Could you check a few things on this model? Use its own coordinates, in mm. A direction names the side the tool comes from. Round coordinates to 2 decimals unless told otherwise and drop trailing zeros. Loops run counter-clockwise (first coordinate to the right, second up) from the corner with the lowest first, then second, coordinate; pieces in that order, holes last. Notation, with made-up numbers: (-19, -2.5) - (-3, -2.5) arc R18 ccw to (-3, 31.5) - close; hole circle Ø10 at (57.25, 86.5). An arc over 180 degrees is marked (long way). Use one line per item in the form item = value.
```python
from build123d import *

# Parameters (mm, degrees)
F0_W      = 30
F0_H      = 22
F1_DEPTH  = 5
F2_DEPTH  = 39.1
F3_W      = 30
F3_H      = 12.7
F4_DEPTH  = 50
F8_W      = 30
F8_H      = 5
F9_DEPTH  = 25
F10_W     = 30
F10_H     = 5
F11_DEPTH = 5
F12_W     = 30
F12_H     = 5
F13_DEPTH = 25
F15_DEPTH = 25
F16_DEPTH = 3
F18_DEPTH = 3
F19_DEPTH = 3
F21_DEPTH = 3
F23_DEPTH = 30
F24_R     = 2.75
F25_DEPTH = 500
F26_W     = 68.0921077728
F26_H     = 72.8289508261
F27_DEPTH = 25
F29_DEPTH = 36
F30_R     = 4.99999
F32_DEPTH = 1
F33_W     = 82.302633673
F33_H     = 75.4934260622
F34_DEPTH = 50


# Not quite as in the source:
# - a fillet or chamfer is up to 0.001 mm smaller than in the source, because OpenCascade refuses the exact size


with BuildPart() as f1:
    # F0 (on Front) → F1 (new body)
    with BuildSketch(Plane.XZ):
        with Locations((0, 7.15)):
            Rectangle(F0_W, F0_H)
        with BuildLine():
            ThreePointArc((-6, -1.7), (-7.7, 0), (-6, 1.7))
            Line((-6, 1.7), (6, 1.7))
            ThreePointArc((6, 1.7), (7.7, 0), (6, -1.7))
            Line((6, -1.7), (-6, -1.7))
        make_face(mode=Mode.SUBTRACT)
        with BuildLine():
            ThreePointArc((-6, 12.6), (-7.7, 14.3), (-6, 16))
            Line((-6, 16), (6, 16))
            ThreePointArc((6, 16), (7.7, 14.3), (6, 12.6))
            Line((6, 12.6), (-6, 12.6))
        make_face(mode=Mode.SUBTRACT)
    extrude(amount=F1_DEPTH)

    # F2 (add): a face of the model
    f2_faces = [f1.faces().sort_by_distance(p)[0] for p in [
        (0, -2.5, 18.15),
    ]]
    extrude(f2_faces, amount=F2_DEPTH)

    # F3 (on face) → F4 (join)
    with BuildSketch(Plane.XZ.offset(5)):
        with Locations((0, 50.9)):
            Rectangle(F3_W, F3_H)
    extrude(amount=F4_DEPTH)

    # F6 (on offset) → F7 (revolve, cut)
    with BuildSketch(Plane.XZ.offset(38.3)):
        Polygon((8, 57.25), (0, 57.25), (0, 44.55), (8, 44.55), (8, 49.05), (4.5, 49.05), (4.5, 53.55), (8, 53.55), align=None)
    revolve(axis=Axis((0, -38.3, 50.9), (0, 0, 1)), mode=Mode.SUBTRACT)

    # F8 (on face) → F9 (join)
    with BuildSketch(Plane(origin=(0, 0, 0), x_dir=(-1, 0, 0), z_dir=(0, 1, 0))):
        with Locations((0, 36.45)):
            Rectangle(F8_W, F8_H)
    extrude(amount=F9_DEPTH)

    # F10 (on face) → F11 (join)
    with BuildSketch(Plane(origin=(0, 0, 33.95), x_dir=(1, 0, 0), z_dir=(0, 0, -1))):
        with Locations((0, -22.5)):
            Rectangle(F10_W, F10_H)
    extrude(amount=F11_DEPTH)

    # F12 (on face) → F13 (join)
    with BuildSketch(Plane(origin=(0, 25, 0), x_dir=(-1, 0, 0), z_dir=(0, 1, 0))):
        with Locations((0, 31.45)):
            Rectangle(F12_W, F12_H)
    extrude(amount=F13_DEPTH)

    # F14 (on face) → F15 (cut)
    with BuildSketch(Plane.XY.offset(33.95)):
        with BuildLine():
            ThreePointArc((7.4548611111, 38.3216117173), (0, 45), (-7.4548611111, 38.3216117173))
            ThreePointArc((-7.4548611111, 38.3216117173), (-10.75, 37.5), (-7.4548611111, 36.6783882827))
            ThreePointArc((-7.4548611111, 36.6783882827), (0, 30), (7.4548611111, 36.6783882827))
            ThreePointArc((7.4548611111, 36.6783882827), (10.75, 37.5), (7.4548611111, 38.3216117173))
        make_face()
    extrude(amount=-F15_DEPTH, mode=Mode.SUBTRACT)

    # F16 (add): a face of the model
    f16_faces = [f1.faces().sort_by_distance(p)[0] for p in [
        (15, -2.5, -2.6351662665),
    ]]
    extrude(f16_faces, amount=F16_DEPTH)

    # F17 (on face) → F18 (join)
    with BuildSketch(Plane.YZ.offset(18)):
        Polygon((50, 33.95), (0, 57.25), (0, 38.95), (25, 38.95), (25, 33.95), align=None)
    extrude(amount=-F18_DEPTH)

    # F19 (add): a face of the model
    f19_faces = [f1.faces().sort_by_distance(p)[0] for p in [
        (-15, -2.5, -2.6351662665),
    ]]
    extrude(f19_faces, amount=F19_DEPTH)

    # F20 (on face) → F21 (join)
    with BuildSketch(Plane(origin=(-18, 0, 0), x_dir=(0, -1, 0), z_dir=(-1, 0, 0))):
        Polygon((0, 57.25), (-50, 33.95), (-25, 33.95), (-25, 38.95), (0, 38.95), align=None)
    extrude(amount=-F21_DEPTH)

    # F22 (on face) → F23 (join, through all)
    with BuildSketch(Plane(origin=(15, 0, 0), x_dir=(0, -1, 0), z_dir=(-1, 0, 0))):
        Polygon((-25, 45.6), (-25, 38.95), (0, 38.95), (0, 57.25), align=None)
    extrude(amount=F23_DEPTH)

    # F24 (on face) → F25 (cut)
    with BuildSketch(Plane.XZ.offset(55)):
        with Locations((-11.1628601777, 51.5)):
            Circle(F24_R)
        with Locations((10.8371398223, 51.5)):
            Circle(F24_R)
    extrude(amount=-F25_DEPTH, mode=Mode.SUBTRACT)

    # F26 (on offset) → F27 (cut)
    with BuildSketch(Plane.XZ.offset(38.3)):
        with Locations((0.2960525453, 29.3092119973)):
            Rectangle(F26_W, F26_H)
    extrude(amount=F27_DEPTH, mode=Mode.SUBTRACT)

    # F28 (on face) → F29 (join)
    with BuildSketch(Plane(origin=(-18, 0, 0), x_dir=(0, -1, 0), z_dir=(-1, 0, 0))):
        Polygon((5, 44.55), (5, 20.35), (16.9268529862, 44.55), align=None)
    extrude(amount=-F29_DEPTH)

    # F30 (radius 5 in the source; OpenCascade refuses exactly that, so slightly less here)
    f30_edges = [f1.edges().sort_by_distance(p)[0] for p in [
        (0, -16.926853, 44.55),
        (0, 20, 33.95),
        (0, -5, 20.35),
    ]]
    fillet(f30_edges, radius=F30_R)

    # F31 (on face) → F32 (cut)
    with BuildSketch(Plane(origin=(-18, 0, 0), x_dir=(0, -1, 0), z_dir=(-1, 0, 0))):
        with BuildLine():
            ThreePointArc((2.083333126, 43.103029569), (2.7667506365, 41.4531137462), (4.4166664593, 40.7696962357))
            Line((4.4166664593, 40.7696962357), (11.4166664593, 40.7696962357))
            ThreePointArc((11.4166664593, 40.7696962357), (13.0665822821, 41.4531137462), (13.7499997926, 43.103029569))
            Line((13.7499997926, 43.103029569), (13.7499997926, 50.103029569))
            ThreePointArc((13.7499997926, 50.103029569), (13.0665822821, 51.7529453918), (11.4166664593, 52.4363629023))
            Line((11.4166664593, 52.4363629023), (4.4166664593, 52.4363629023))
            ThreePointArc((4.4166664593, 52.4363629023), (2.7667506365, 51.7529453918), (2.083333126, 50.103029569))
            Line((2.083333126, 50.103029569), (2.083333126, 43.103029569))
        make_face()
        with BuildLine():
            Line((9.6666664593, 43.103029569), (6.1666664593, 43.103029569))
            ThreePointArc((6.1666664593, 43.103029569), (4.9292295922, 43.6155927019), (4.4166664593, 44.853029569))
            Line((4.4166664593, 44.853029569), (4.4166664593, 48.353029569))
            ThreePointArc((4.4166664593, 48.353029569), (4.9292295922, 49.5904664361), (6.1666664593, 50.103029569))
            Line((6.1666664593, 50.103029569), (9.6666664593, 50.103029569))
            ThreePointArc((9.6666664593, 50.103029569), (10.9041033264, 49.5904664361), (11.4166664593, 48.353029569))
            Line((11.4166664593, 48.353029569), (11.4166664593, 44.853029569))
            ThreePointArc((11.4166664593, 44.853029569), (11.3861769533, 44.5277855668), (11.2957708468, 44.2138747406))
            Line((11.2957708593, 44.2138747357), (8.8241202093, 46.6855253857))
            ThreePointArc((8.8241201983, 46.6855253747), (8.4116412426, 46.8563797523), (7.9991622869, 46.6855253747))
            Line((7.999162276, 46.6855253857), (7.9166664593, 46.603029569))
            Line((7.9166664593, 46.603029569), (7.8341706426, 46.5205337523))
            ThreePointArc((7.8341706536, 46.5205337413), (7.663316276, 46.1080547857), (7.8341706536, 45.69557583))
            Line((7.8341706426, 45.695575819), (10.3058212926, 43.223925169))
            ThreePointArc((10.3058212877, 43.2239251815), (9.9919104615, 43.133519075), (9.6666664593, 43.103029569))
        make_face(mode=Mode.SUBTRACT)
    extrude(amount=-F32_DEPTH, mode=Mode.SUBTRACT)

    # F33 (on face) → F34 (cut)
    with BuildSketch(Plane(origin=(0, 50, 0), x_dir=(-1, 0, 0), z_dir=(0, 1, 0))):
        with Locations((4.7368425876, 23.2401336543)):
            Rectangle(F33_W, F33_H)
        Polygon((-18, 33.95), (-15, 33.95), (15, 33.95), (18, 33.95), (18, 28.95), (-18, 28.95), align=None, mode=Mode.SUBTRACT)
        Polygon((15, 33.95), (-15, 33.95), (-18, 33.95), (-18, 28.95), (18, 28.95), (18, 33.95), align=None)
    extrude(amount=-F34_DEPTH, mode=Mode.SUBTRACT)


solid = f1.part
```
1. Please list where these lines run through material, in increasing order: line 1 along X through (y, z) = (-14, 51); line 2 along Z through (x, y) = (-3.5, -35); line 3 along Y through (x, z) = (10, 4).
Solution:
line_1 = -18 to -13.87, -8.46 to 8.13, 13.54 to 18
line_2 = 49.05 to 53.55
line_3 = -5 to 0
2. We'd pull the mould along X, two halves only. Please class faces 5 (the face through (18, -15, 41)), 6 (the face through (-11.521, -19.418, 54.227)), 7 (the face through (7.7, -2.5, 0)), 8 (the face through (-18, -12, 36)): +X half, -X half, draft (parallel to the pull), parting line (faces both ways), or undercut.
Solution:
face_5 = +X half
face_6 = undercut
face_7 = undercut
face_8 = -X half
3. For P1, Ø1, axis at x = 2.5, y = -34, coming from the -Z side; P2, Ø0.5, axis at x = -17.5, y = -7, coming from the -Z side; P3, Ø1, axis at x = 5, y = -32, coming from the -Z side; P4, Ø4.5, axis at x = -11.16, z = 51.5, coming from the +Y side, each with a flat end and sliding along its axis, tell me the tip position at first contact or that it passes through.
Solution:
P1 = 49.05
P2 = 23.9
P3 = 44.55
P4 = through
4. On a 3-axis mill with a long thin cutter (end or side, diameter ignored), from which of +Z, -Z, +X, -X, +Y, -Y can I reach the whole of each face in a straight line? I mean faces 1 (the face through (-17.51, -4.92, 49.58)), 2 (the face through (0, -33, 53.55)), 3 (the face through (-7.7, -2.5, 14.3)), 4 (the face through (0.176, -30.302, 46.832)). Say none if no direction works.
Solution:
face_1 = -X
face_2 = +Z, -Y
face_3 = +Y, -Y
face_4 = -Z, -Y
5. If we section it at D-D, the plane z = 51.5: Write out the boundary of the cut face in (x, y), plus the area to 3 significant figures.
Solution:
outline = (-18, -38.3) - (-13.91, -38.3) - (-13.91, 0) - (-18, 0) - (-18, -2.55) - (-17, -2.55) - (-17, -13.29) - (-18, -13.29) - close; (-8.41, -38.3) - (-4.5, -38.3) arc R4.5 cw to (4.5, -38.3) - (8.09, -38.3) - (8.09, 0) - (-8.41, 0) - close; (13.59, -38.3) - (18, -38.3) - (18, 0) - (13.59, 0) - close
area = 915 mm^2
6. If we section it at B-B, the plane x = 0: Write out the boundary of the cut face in (y, z).
Solution:
outline = (-33.8, 49.05) - (-30.3, 49.05) - (-30.3, 44.55) - (-20.04, 44.55) arc R5 cw to (-15.55, 41.76) - (-5.52, 21.4) arc R5 cw to (-5, 19.18) - (-5, 16) - (0, 16) - (0, 57.25) - (-30.3, 57.25) - (-30.3, 53.55) - (-33.8, 53.55) - close; (-5, -3.85) - (0, -3.85) - (0, -1.7) - (-5, -1.7) - close; (-5, 1.7) - (0, 1.7) - (0, 12.6) - (-5, 12.6) - close
7. If we section it at C-C, the plane y = -29: Write out the boundary of the cut face in (x, z).
Solution:
outline = (-18, 44.55) - (18, 44.55) - (18, 57.25) - (-18, 57.25) - close; hole circle Ø5.5 at (-11.16, 51.5); hole circle Ø5.5 at (10.84, 51.5)
8. If we section it at A-A, the plane z = 0: Write out the boundary of the cut face in (x, y), plus the area to 3 significant figures.
Solution:
outline = (-18, -5) - (-7.7, -5) - (-7.7, 0) - (-18, 0) - close; (7.7, -5) - (18, -5) - (18, 0) - (7.7, 0) - close
area = 103 mm^2
